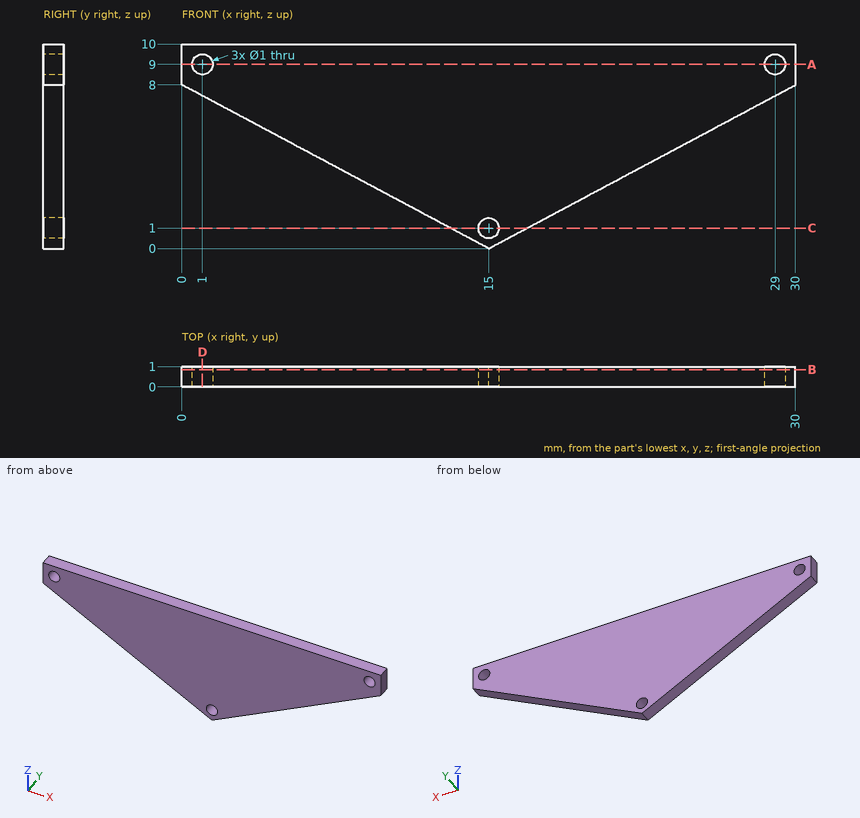
The drawing under review shows one solid part. Ordinate dimensions are in mm from its lowest x, y, z. Coordinates: 2 decimals unless noted, no trailing zeros. Write each loop counter-clockwise with the first axis right and the second up, starting at its lowest first coordinate (ties: lowest second). Pieces come first, ordered by that corner, then holes. Notation, with made-up numbers: (31, -40) - (39, -40) arc R15 cw to (39, -21) - close; hole circle Ø2 at (39.5, 62). An arc over 180 degrees is marked (long way). Use one line per item in the form item = value.
Q1. Consider section D-D (x = 1). Write out the cut boundary in (y, z).
Taken from the geometry:
outline = (0, 7.47) - (1, 7.47) - (1, 8.5) - (0, 8.5) - close; (0, 9.5) - (1, 9.5) - (1, 10) - (0, 10) - close
Q2. Consider section B-B (y = 0.85). Write out the cut boundary in (x, z).
Taken from the geometry:
outline = (0, 8) - (15, 0) - (30, 8) - (30, 10) - (0, 10) - close; hole circle Ø1 at (1, 9); hole circle Ø1 at (15, 1); hole circle Ø1 at (29, 9)
Q3. For probe 1 along Z at (x, y) = (1, 0.3); probe 2 along X at (y, z) = (0.25, 6.75); probe 3 along Z at (x, y) = (8, 0.15), list the stretches that pass through material, from the lowest coordinate up.
Taken from the geometry:
probe_1 = 7.47 to 8.5, 9.5 to 10
probe_2 = 2.34 to 27.66
probe_3 = 3.73 to 10
Q4. Consider section C-C (z = 1). Write out the cut boundary in (x, y) (3 decimals), plus the area to 3 significant figures.
Taken from the geometry:
outline = (13.125, 0) - (14.5, 0) - (14.5, 1) - (13.125, 1) - close; (15.5, 0) - (16.875, 0) - (16.875, 1) - (15.5, 1) - close
area = 2.75 mm^2
Q5. Consider section A-A (z = 9). Write out the cut boundary in (x, y).
Taken from the geometry:
outline = (0, 0) - (0.5, 0) - (0.5, 1) - (0, 1) - close; (1.5, 0) - (28.5, 0) - (28.5, 1) - (1.5, 1) - close; (29.5, 0) - (30, 0) - (30, 1) - (29.5, 1) - close
